from build123d import *

# Parameters (mm, degrees)
F0_W     = 0.4
F0_H     = 1
F0_W_2   = 1
F1_DEPTH = 5


with BuildPart() as f1:
    # F0 (on Top) → F1 (new body)
    with BuildSketch(Plane.XY):
        Polygon((28.977659, 27.887268), (-21.822341, 27.887268), (-21.822341, -13.112732), (-21.422341, -13.112732), (-21.422341, 26.887268), (-20.422341, 26.887268), (-20.422341, -13.112732), (-20.022341, -13.112732), (-20.022341, 26.887268), (-19.022341, 26.887268), (-19.022341, -13.112732), (-18.622341, -13.112732), (-18.622341, 26.887268), (-17.622341, 26.887268), (-17.622341, -13.112732), (-17.222341, -13.112732), (-17.222341, 26.887268), (-16.222341, 26.887268), (-16.222341, -13.112732), (-15.822341, -13.112732), (-15.822341, 26.887268), (-14.822341, 26.887268), (-14.822341, -13.112732), (-14.422341, -13.112732), (-14.422341, 26.887268), (-13.422341, 26.887268), (-13.422341, -13.112732), (-13.022341, -13.112732), (-13.022341, 26.887268), (-12.022341, 26.887268), (-12.022341, -13.112732), (-11.622341, -13.112732), (-11.622341, 26.887268), (-10.622341, 26.887268), (-10.622341, -13.112732), (-10.222341, -13.112732), (-10.222341, 26.887268), (-9.222341, 26.887268), (-9.222341, -13.112732), (-8.822341, -13.112732), (-8.822341, 26.887268), (-7.822341, 26.887268), (-7.822341, -13.112732), (-7.422341, -13.112732), (-7.422341, 26.887268), (-6.422341, 26.887268), (-6.422341, -13.112732), (-6.022341, -13.112732), (-6.022341, 26.887268), (-5.022341, 26.887268), (-5.022341, -13.112732), (-4.622341, -13.112732), (-4.622341, 26.887268), (-3.622341, 26.887268), (-3.622341, -13.112732), (-3.222341, -13.112732), (-3.222341, 26.887268), (-2.222341, 26.887268), (-2.222341, -13.112732), (-1.822341, -13.112732), (-1.822341, 26.887268), (-0.822341, 26.887268), (-0.822341, -13.112732), (-0.422341, -13.112732), (-0.422341, 26.887268), (0.577659, 26.887268), (0.577659, -13.112732), (0.977659, -13.112732), (0.977659, 26.887268), (1.977659, 26.887268), (1.977659, -13.112732), (2.377659, -13.112732), (2.377659, 26.887268), (3.377659, 26.887268), (3.377659, -13.112732), (3.777659, -13.112732), (3.777659, 26.887268), (4.777659, 26.887268), (4.777659, -13.112732), (5.177659, -13.112732), (5.177659, 26.887268), (6.177659, 26.887268), (6.177659, -13.112732), (6.577659, -13.112732), (6.577659, 26.887268), (7.577659, 26.887268), (7.577659, -13.112732), (7.977659, -13.112732), (7.977659, 26.887268), (8.977659, 26.887268), (8.977659, -13.112732), (9.377659, -13.112732), (9.377659, 26.887268), (10.377659, 26.887268), (10.377659, -13.112732), (10.777659, -13.112732), (10.777659, 26.887268), (11.777659, 26.887268), (11.777659, -13.112732), (12.177659, -13.112732), (12.177659, 26.887268), (13.177659, 26.887268), (13.177659, -13.112732), (13.577659, -13.112732), (13.577659, 26.887268), (14.577659, 26.887268), (14.577659, -13.112732), (14.977659, -13.112732), (14.977659, 26.887268), (15.977659, 26.887268), (15.977659, -13.112732), (16.377659, -13.112732), (16.377659, 26.887268), (17.377659, 26.887268), (17.377659, -13.112732), (17.777659, -13.112732), (17.777659, 26.887268), (18.777659, 26.887268), (18.777659, -13.112732), (19.177659, -13.112732), (19.177659, 26.887268), (20.177659, 26.887268), (20.177659, -13.112732), (20.577659, -13.112732), (20.577659, 26.887268), (21.577659, 26.887268), (21.577659, -13.112732), (21.977659, -13.112732), (21.977659, 26.887268), (22.977659, 26.887268), (22.977659, -13.112732), (23.377659, -13.112732), (23.377659, 26.887268), (24.377659, 26.887268), (24.377659, -13.112732), (24.777659, -13.112732), (24.777659, 26.887268), (25.777659, 26.887268), (25.777659, -13.112732), (26.177659, -13.112732), (26.177659, 26.887268), (27.177659, 26.887268), (27.177659, -13.112732), (27.577659, -13.112732), (27.577659, 26.887268), (28.577659, 26.887268), (28.577659, -13.112732), (28.577659, -14.112732), (28.977659, -14.112732), (28.977659, 26.887268), align=None)
        with Locations((-21.622341, -13.612732)):
            Rectangle(F0_W, F0_H)
        with Locations((-20.922341, -13.612732)):
            Rectangle(F0_W_2, F0_H)
        with Locations((-20.222341, -13.612732)):
            Rectangle(F0_W, F0_H)
        with Locations((-19.522341, -13.612732)):
            Rectangle(F0_W_2, F0_H)
        with Locations((28.077659, -13.612732)):
            Rectangle(F0_W_2, F0_H)
        with Locations((-18.822341, -13.612732)):
            Rectangle(F0_W, F0_H)
        with Locations((27.377659, -13.612732)):
            Rectangle(F0_W, F0_H)
        with Locations((-18.122341, -13.612732)):
            Rectangle(F0_W_2, F0_H)
        with Locations((26.677659, -13.612732)):
            Rectangle(F0_W_2, F0_H)
        with Locations((-17.422341, -13.612732)):
            Rectangle(F0_W, F0_H)
        with Locations((25.977659, -13.612732)):
            Rectangle(F0_W, F0_H)
        with Locations((-16.722341, -13.612732)):
            Rectangle(F0_W_2, F0_H)
        with Locations((25.277659, -13.612732)):
            Rectangle(F0_W_2, F0_H)
        with Locations((-16.022341, -13.612732)):
            Rectangle(F0_W, F0_H)
        with Locations((24.577659, -13.612732)):
            Rectangle(F0_W, F0_H)
        with Locations((-15.322341, -13.612732)):
            Rectangle(F0_W_2, F0_H)
        with Locations((23.877659, -13.612732)):
            Rectangle(F0_W_2, F0_H)
        with Locations((-14.622341, -13.612732)):
            Rectangle(F0_W, F0_H)
        with Locations((23.177659, -13.612732)):
            Rectangle(F0_W, F0_H)
        with Locations((-13.922341, -13.612732)):
            Rectangle(F0_W_2, F0_H)
        with Locations((22.477659, -13.612732)):
            Rectangle(F0_W_2, F0_H)
        with Locations((-13.222341, -13.612732)):
            Rectangle(F0_W, F0_H)
        with Locations((21.777659, -13.612732)):
            Rectangle(F0_W, F0_H)
        with Locations((-12.522341, -13.612732)):
            Rectangle(F0_W_2, F0_H)
        with Locations((21.077659, -13.612732)):
            Rectangle(F0_W_2, F0_H)
        with Locations((-11.822341, -13.612732)):
            Rectangle(F0_W, F0_H)
        with Locations((20.377659, -13.612732)):
            Rectangle(F0_W, F0_H)
        with Locations((-11.122341, -13.612732)):
            Rectangle(F0_W_2, F0_H)
        with Locations((19.677659, -13.612732)):
            Rectangle(F0_W_2, F0_H)
        with Locations((-10.422341, -13.612732)):
            Rectangle(F0_W, F0_H)
        with Locations((18.977659, -13.612732)):
            Rectangle(F0_W, F0_H)
        with Locations((-9.722341, -13.612732)):
            Rectangle(F0_W_2, F0_H)
        with Locations((18.277659, -13.612732)):
            Rectangle(F0_W_2, F0_H)
        with Locations((-9.022341, -13.612732)):
            Rectangle(F0_W, F0_H)
        with Locations((17.577659, -13.612732)):
            Rectangle(F0_W, F0_H)
        with Locations((-8.322341, -13.612732)):
            Rectangle(F0_W_2, F0_H)
        with Locations((16.877659, -13.612732)):
            Rectangle(F0_W_2, F0_H)
        with Locations((-7.622341, -13.612732)):
            Rectangle(F0_W, F0_H)
        with Locations((16.177659, -13.612732)):
            Rectangle(F0_W, F0_H)
        with Locations((-6.922341, -13.612732)):
            Rectangle(F0_W_2, F0_H)
        with Locations((15.477659, -13.612732)):
            Rectangle(F0_W_2, F0_H)
        with Locations((-6.222341, -13.612732)):
            Rectangle(F0_W, F0_H)
        with Locations((14.777659, -13.612732)):
            Rectangle(F0_W, F0_H)
        with Locations((-5.522341, -13.612732)):
            Rectangle(F0_W_2, F0_H)
        with Locations((14.077659, -13.612732)):
            Rectangle(F0_W_2, F0_H)
        with Locations((-4.822341, -13.612732)):
            Rectangle(F0_W, F0_H)
        with Locations((13.377659, -13.612732)):
            Rectangle(F0_W, F0_H)
        with Locations((-4.122341, -13.612732)):
            Rectangle(F0_W_2, F0_H)
        with Locations((12.677659, -13.612732)):
            Rectangle(F0_W_2, F0_H)
        with Locations((-3.422341, -13.612732)):
            Rectangle(F0_W, F0_H)
        with Locations((11.977659, -13.612732)):
            Rectangle(F0_W, F0_H)
        with Locations((-2.722341, -13.612732)):
            Rectangle(F0_W_2, F0_H)
        with Locations((11.277659, -13.612732)):
            Rectangle(F0_W_2, F0_H)
        with Locations((-2.022341, -13.612732)):
            Rectangle(F0_W, F0_H)
        with Locations((10.577659, -13.612732)):
            Rectangle(F0_W, F0_H)
        with Locations((-1.322341, -13.612732)):
            Rectangle(F0_W_2, F0_H)
        with Locations((9.877659, -13.612732)):
            Rectangle(F0_W_2, F0_H)
        with Locations((-0.622341, -13.612732)):
            Rectangle(F0_W, F0_H)
        with Locations((9.177659, -13.612732)):
            Rectangle(F0_W, F0_H)
        with Locations((0.077659, -13.612732)):
            Rectangle(F0_W_2, F0_H)
        with Locations((8.477659, -13.612732)):
            Rectangle(F0_W_2, F0_H)
        with Locations((0.777659, -13.612732)):
            Rectangle(F0_W, F0_H)
        with Locations((7.777659, -13.612732)):
            Rectangle(F0_W, F0_H)
        with Locations((1.477659, -13.612732)):
            Rectangle(F0_W_2, F0_H)
        with Locations((7.077659, -13.612732)):
            Rectangle(F0_W_2, F0_H)
        with Locations((2.177659, -13.612732)):
            Rectangle(F0_W, F0_H)
        with Locations((6.377659, -13.612732)):
            Rectangle(F0_W, F0_H)
        with Locations((2.877659, -13.612732)):
            Rectangle(F0_W_2, F0_H)
        with Locations((5.677659, -13.612732)):
            Rectangle(F0_W_2, F0_H)
        with Locations((3.577659, -13.612732)):
            Rectangle(F0_W, F0_H)
        with Locations((4.977659, -13.612732)):
            Rectangle(F0_W, F0_H)
        with Locations((4.277659, -13.612732)):
            Rectangle(F0_W_2, F0_H)
    extrude(amount=F1_DEPTH)


solid = f1.part
Here's how the part is built. I have some questions about the finished solid (model axes, mm). Coordinates: 2 decimals unless noted, no trailing zeros.
Item 1: If I drill on line 1 (Y direction, x = 7.5, z = 3.75), over which ranges is the centre line in solid material (lowest first)?
Item 2: If we mould it in two halves opening along X, with no side actions, what happens to faces 1 (the flat face through (28, 26.887, 2)), 2 (the flat face through (-16.222, 7, 2)), 3 (the flat face through (28.978, 7, 2))? For each: +X half, -X half, draft (parallel to the pull), parting line (faces both ways), or undercut.
Item 3: I want a section at A-A on y = 17. Count the separate pieces of the cut face and the enclosed holes in it, and give its area (3 significant figures).
Findings below:
1. line 1: y = -14.11 to -13.11, 26.89 to 27.89
2. face 1: undercut
2. face 2: undercut
2. face 3: +X half
3. separate pieces: 37
3. enclosed holes: 0
3. area: 74.0 mm2
